Check sheet for the modelled part. Datum: model origin and axes. Units: mm. Face numbers are marked on the shaded views. A direction names the side the tool comes from. Round coordinates to 2 decimals unless told otherwise and drop trailing zeros. Loops run counter-clockwise (first coordinate to the right, second up) from the corner with the lowest first, then second, coordinate; pieces in that order, holes last. Notation, with made-up numbers: M 32,-19 L 73,-19 A23 ccw 73,1 Z; hole C 21,31 d7. An arc over 180 degrees is marked long. Write item = value, one per line. Start each with the question number.
(1) Cross-section at C-C on y = -39.85. Record the boundary of the cut face in (x, z), plus the area to 4 significant figures.
(2) Go/stop test with flat-tipped pins: P1, Ø1.6, axis at y = -39, z = 93.5, coming from the -X side; P2, Ø1.8, axis at y = -39.85, z = 92.9, coming from the +X side; P3, Ø10, axis at x = 10, z = 58.5, coming from the -Y side; P4, Ø0.8, axis at x = -5.5, y = -30.5, coming from the -Z side. Record where each tip stops, or that it passes through.
(3) Cross-section at D-D on x = 6.75. Record the boundary of the cut face in (y, z), plus the area to 3 significant figures.
(4) Set-up check for the marked faces 1, 2 and 3: record each of +Z, -Z, +X, -X, +Y, -Y from which the full face is reachable in a straight line by a thin tool's end or side.
(5) Scan lines: L1, parallel to Z at x = 6.25, y = -29.85; L2, parallel to Y at x = 8, z = 44.3; L3, parallel to Z at x = -2.5, y = -42.5. Record each from-to range of solid material in increasing order. Write a range as from..to.
(6) Cross-section at B-B on z = 76. Record the boundary of the cut face in (x, y), plus the area to 3 significant figures.
(7) Mould release check, pull along Z, two halves, no side actions. Record for the marked faces 4, 5, 6 and 7: pulls with the +Z half, pulls with the -Z half, needs draft (parallel to the pull), parting line crosses it, or undercut.
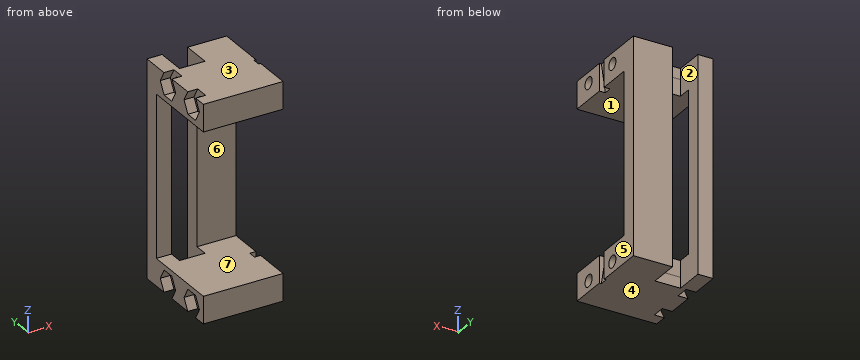
from build123d import *

# Parameters (mm, degrees)
SKETCH050_R             = 1.5
PAD021_DEPTH            = 20
POCKET001_DEPTH         = 27.001
POCKET001_DEPTH_BACK    = 27.001
POCKET032_DEPTH         = 1
POCKET033_DEPTH         = 2.5
SKETCH008_W             = 54
SKETCH008_H             = 1.25
POCKET003_DEPTH         = 0.001
POCKET003_DEPTH_BACK    = 20.001
BODY009_PITCH_ANGLE     = 90
BODY009_PLACEMENT_ANGLE = 90


with BuildPart() as part:
    # Sketch050 → Pad021 (new body)
    with BuildSketch(Plane.XZ):
        Polygon((-27, 25), (27, 25), (27, 0), (20.2, 0), (20.2, 19.8), (20, 19.8), (-20, 19.8), (-20.2, 19.8), (-20.2, 0), (-27, 0), align=None)
        with Locations((24.3, 14.9)):
            Circle(SKETCH050_R, mode=Mode.SUBTRACT)
        with Locations((24.3, 4.9)):
            Circle(SKETCH050_R, mode=Mode.SUBTRACT)
        with Locations((-24.3, 14.9)):
            Circle(SKETCH050_R, mode=Mode.SUBTRACT)
        with Locations((-24.3, 4.9)):
            Circle(SKETCH050_R, mode=Mode.SUBTRACT)
    extrude(amount=PAD021_DEPTH)

    # Sketch007 → Pocket001 (cut, two sides)
    with BuildSketch(Plane.YZ) as pocket001_sk:
        Polygon((-10.2, 16.4), (-10.2, 23.75), (-7.25, 23.75), (-6.749999, 23.75), (-3.8, 23.75), (-3.8, 16.4), align=None)
    extrude(amount=-POCKET001_DEPTH, mode=Mode.SUBTRACT)
    extrude(pocket001_sk.sketch, amount=POCKET001_DEPTH_BACK, mode=Mode.SUBTRACT)

    # Sketch003 → Pocket032 (cut, symmetric)
    with BuildSketch(Plane(origin=(0, -23.75, 10.448022), x_dir=(1, 0, 0), z_dir=(0, 0, -1))):
        Polygon((-20.2, -3.75), (-27, -3.75), (-27, -4.25), (-20.2, -5.25), align=None)
        Polygon((20.2, -3.75), (27, -3.75), (27, -4.25), (20.2, -5.25), align=None)
    extrude(amount=POCKET032_DEPTH, both=True, mode=Mode.SUBTRACT)

    # Sketch051 → Pocket033 (cut)
    with BuildSketch(Plane.XZ):
        Polygon((-27.1, 16.516581), (-27.1, 13.283419), (-24.3, 11.666838), (-21.5, 13.283419), (-21.5, 16.516581), (-24.3, 18.133162), align=None)
        Polygon((-27.1, 6.516581), (-27.1, 3.283419), (-24.3, 1.666838), (-21.5, 3.283419), (-21.5, 6.516581), (-24.3, 8.133162), align=None)
        Polygon((21.5, 16.516581), (21.5, 13.283419), (24.3, 11.666838), (27.1, 13.283419), (27.1, 16.516581), (24.3, 18.133162), align=None)
        Polygon((21.5, 6.516581), (21.5, 3.283419), (24.3, 1.666838), (27.1, 3.283419), (27.1, 6.516581), (24.3, 8.133162), align=None)
    extrude(amount=POCKET033_DEPTH, mode=Mode.SUBTRACT)

    # Sketch008 → Pocket003 (cut, two sides)
    with BuildSketch(Plane.XZ) as pocket003_sk:
        with Locations((0, 24.375)):
            Rectangle(SKETCH008_W, SKETCH008_H)
    extrude(amount=-POCKET003_DEPTH, mode=Mode.SUBTRACT)
    extrude(pocket003_sk.sketch, amount=POCKET003_DEPTH_BACK, mode=Mode.SUBTRACT)


with BuildPart() as part_1:
    # Body009 pitch: moved
    add(part.part.rotate(Axis((0, 0, 0), (0, 1, 0)), BODY009_PITCH_ANGLE))


with BuildPart() as part_2:
    # Body009 placement: moved
    add(part_1.part.moved(Location((-7.4, -44.75, 68.6))).rotate(Axis((-7.4, -44.75, 68.6), (0, 0, 1)), BODY009_PLACEMENT_ANGLE))


solid = part_2.part
Result:
q1.outline = M -7.4,47.1 L -4.9,47.1 L -4.9,45.8 L 12.6,45.8 L 12.6,48.4 L -7.4,48.4 Z; M -7.4,88.8 L 12.6,88.8 L 12.6,91.4 L -4.9,91.4 L -4.9,90.1 L -7.4,90.1 Z; M -4.9,41.6 L 12.6,41.6 L 12.6,42.8 L -4.9,42.8 Z; M -4.9,94.4 L 12.6,94.4 L 12.6,95.6 L -4.9,95.6 Z
q1.area = 139.5 mm^2
q2.P1 = -4.9
q2.P2 = through
q2.P3 = -24.95
q2.P4 = 47.1
q3.outline = M -44.75,41.6 L -21,41.6 L -21,95.6 L -44.75,95.6 L -44.75,88.8 L -24.95,88.8 L -24.95,48.4 L -44.75,48.4 Z; hole C -39.85,44.3 d3; hole C -39.85,92.9 d3; hole C -29.85,44.3 d3; hole C -29.85,92.9 d3
q3.area = 454 mm^2
q4.face_1 = +X, -X, -Y
q4.face_2 = +Z, -Z, +Y
q4.face_3 = +Z, +X, -X, +Y, -Y
q5.L1 = 41.6..42.8, 45.8..48.4, 88.8..91.4, 94.4..95.6
q5.L2 = -44.75..-41.35, -38.35..-31.35, -28.35..-21
q5.L3 = 41.6..48.4, 88.8..95.6
q6.outline = M -7.4,-24.95 L -3.6,-24.95 L -3.6,-21 L -7.4,-21 Z; M 2.8,-24.95 L 12.6,-24.95 L 12.6,-21 L 2.8,-21 Z
q6.area = 53.7 mm^2
q7.face_4 = pulls with the -Z half
q7.face_5 = needs draft
q7.face_6 = undercut
q7.face_7 = undercut
